from build123d import *

# Parameters (mm, degrees)
SKETCH1_R           = 2
SKETCH1_R_2         = 6
SKETCH1_R_3         = 3
BOSS_EXTRUDE1_DEPTH = 14
SKETCH2_R           = 6
SKETCH2_R_2         = 3
BOSS_EXTRUDE2_DEPTH = 38
SKETCH3_R           = 3
BOSS_EXTRUDE3_DEPTH = 12
SKETCH4_R           = 6
BOSS_EXTRUDE4_DEPTH = 22
CUT_EXTRUDE1_START  = -14
CUT_EXTRUDE1_DEPTH  = 14
CHAMFER1_SIZE       = 1
SKETCH6_R           = 2.5
CUT_EXTRUDE2_DEPTH  = 5
SKETCH7_R           = 1.5
CUT_EXTRUDE3_DEPTH  = 15


with BuildPart() as part:
    # Sketch1 → Boss-Extrude1 (new body)
    with BuildSketch(Plane(origin=(0, 0, 0), x_dir=(1, 0, 0), z_dir=(0, 1, 0))):
        with BuildLine():
            Line((5.196152423, -13), (-5.196152423, -13))
            ThreePointArc((-5.196152423, -13), (0, 14), (5.196152423, -13))
        make_face()
        with Locations(Location((-9, 0, 0), (0, 0, 270))):
            Circle(SKETCH1_R, mode=Mode.SUBTRACT)
        with Locations(Location((9, 0, 0), (0, 0, 270))):
            Circle(SKETCH1_R, mode=Mode.SUBTRACT)
        with Locations(Location((0, 5, 0), (0, 0, 270))):
            Circle(SKETCH1_R_2, mode=Mode.SUBTRACT)
        with Locations(Location((0, -8, 0), (0, 0, 270))):
            Circle(SKETCH1_R_3, mode=Mode.SUBTRACT)
    extrude(amount=BOSS_EXTRUDE1_DEPTH)

    # Sketch2 → Boss-Extrude2 (add)
    with BuildSketch(Plane(origin=(0, 14, 0), x_dir=(1, 0, 0), z_dir=(0, 1, 0))):
        with BuildLine():
            Line((-5.196152423, -13), (5.196152423, -13))
            ThreePointArc((5.196152423, -13), (0, 14), (-5.196152423, -13))
        make_face()
        with Locations(Location((0, 5, 0), (0, 0, 270))):
            Circle(SKETCH2_R, mode=Mode.SUBTRACT)
        with Locations(Location((0, -8, 0), (0, 0, 270))):
            Circle(SKETCH2_R_2, mode=Mode.SUBTRACT)
    extrude(amount=BOSS_EXTRUDE2_DEPTH)

    # Sketch3 → Boss-Extrude3 (add)
    with BuildSketch(Plane(origin=(0, 52, 0), x_dir=(1, 0, 0), z_dir=(0, 1, 0))):
        with BuildLine():
            Line((-5.196152423, -13), (5.196152423, -13))
            ThreePointArc((5.196152423, -13), (0, 14), (-5.196152423, -13))
        make_face()
        with Locations(Location((0, -8, 0), (0, 0, 270))):
            Circle(SKETCH3_R, mode=Mode.SUBTRACT)
    extrude(amount=BOSS_EXTRUDE3_DEPTH)

    # Sketch4 → Boss-Extrude4 (add)
    with BuildSketch(Plane(origin=(0, 64, 0), x_dir=(1, 0, 0), z_dir=(0, 1, 0))):
        with Locations(Location((0, 0, 0), (0, 0, 251.426650281))):
            Circle(SKETCH4_R)
    extrude(amount=BOSS_EXTRUDE4_DEPTH)

    # Sketch5 → Cut-Extrude1 (cut)
    with BuildSketch(Plane(origin=(0, 86, 0), x_dir=(1, 0, 0), z_dir=(0, 1, 0)).offset(CUT_EXTRUDE1_START)):
        with BuildLine():
            Line((5, 3.31662479), (5, -3.31662479))
            ThreePointArc((5, -3.31662479), (6, 0), (5, 3.31662479))
        make_face()
    extrude(amount=CUT_EXTRUDE1_DEPTH, mode=Mode.SUBTRACT)

    # Chamfer1
    chamfer1_edges = [part.edges().sort_by_distance(p)[0] for p in [
        (-4.759608727, 86, -3.653234836),
    ]]
    chamfer(chamfer1_edges, length=CHAMFER1_SIZE - 0.0001)  # a hair under: the kernel refuses the full size

    # Sketch6 → Cut-Extrude2 (cut)
    with BuildSketch(Plane.XY.offset(13)):
        with Locations((0, 31.800606355)):
            Circle(SKETCH6_R)
    extrude(amount=-CUT_EXTRUDE2_DEPTH, mode=Mode.SUBTRACT)

    # Sketch7 → Cut-Extrude3 (cut)
    with BuildSketch(Plane.XY.offset(13)):
        with Locations((0, 55)):
            Circle(SKETCH7_R)
    extrude(amount=-CUT_EXTRUDE3_DEPTH, mode=Mode.SUBTRACT)


solid = part.part
The model under review builds one solid part; all positions refer to its coordinate system, in mm. A direction names the side the tool comes from. Coordinates: 2 decimals unless noted, no trailing zeros. Write each loop counter-clockwise with the first axis right and the second up, starting at its lowest first coordinate (ties: lowest second). Pieces come first, ordered by that corner, then holes. Notation, with made-up numbers: (77, 13) - (94, 13) arc R22 cw to (94, 51) - close; hole circle Ø10 at (82, 77.25). An arc over 180 degrees is marked (long way). Answer as a JSON object with one key per item and string values. Group by question number.
1. Clearance check with flat-ended pins moving along their axes: pin 1 Ø0.9 at (x, y) = (0.5, 55) entering from +Z; pin 2 Ø11 at (x, z) = (0, -5) entering from -Y; pin 3 Ø8 at (x, y) = (-10, 34.5) entering from -Z. State where each tip first meets the part, or that it passes through.
2. Add section D-D (y = 39). Give the boundary of the cut face in (x, z), plus the area to 3 significant figures.
3. Add section B-B (z = 8). Give the boundary of the cut face in (x, y).
4. Mouldability with a two-part tool opening along Y and no side actions: class faces 1 (the face through (0, 52, -5)), 2 (the face through (1.386, 54.425, 11.816)), 3 (the face through (5, 79, 0)) as pulls with the +Y half, pulls with the -Y half, needs draft (parallel to the pull), parting line crosses it, or undercut.
5. Add section C-C (y = 55). Give the boundary of the cut face in (x, z), plus the area to 3 significant figures.
6. Add section A-A (x = 0). Give the number of separate pieces and of enclosed holes in the cut face, plus the area to 3 significant figures.
7. Machinability: for faces 4 (the face through (-5.928, 74.353, 0.929)), 5 (the face through (11, 7, 0)), 6 (the face through (1.386, 54.425, 1.753)), 7 (the face through (0, 86, 0)), which of the approach directions +Z, -Z, +X, -X, +Y, -Y give a long, thin tool a straight path to every point of the face, cutting with its end or side? Answer none if there is none.
8. To check wall thickness, follow probe 1 along Z at (x, y) = (-0.25, 37.5); probe 2 along X at (y, z) = (7.75, 0); probe 3 along Y at (x, z) = (0, 0). State the ranges of each line that lie inside material, in increasing order.
Findings:
{
 "1": {"pin 1": "z = -2", "pin 2": "y = 52", "pin 3": "z = -12.65"},
 "2": {"outline": "(-5.2, 13) arc R14 ccw (long way) to (5.2, 13) - close; hole circle Ø12 at (0, -5); hole circle Ø6 at (0, 8)", "area": "467 mm²"},
 "3": {"outline": "(-11.49, 0) - (-3, 0) - (-3, 64) - (-11.49, 64) - close; (3, 0) - (11.49, 0) - (11.49, 64) - (3, 64) - close"},
 "4": {"face 1": "pulls with the -Y half", "face 2": "undercut", "face 3": "needs draft"},
 "5": {"outline": "(-5.2, 13) arc R14 ccw (long way) to (5.2, 13) - (1.5, 13) - (1.5, 10.6) arc R3 cw to (1.5, 5.4) - (1.5, -2) - (-1.5, -2) - (-1.5, 5.4) arc R3 cw to (-1.5, 10.6) - (-1.5, 13) - close", "area": "553 mm²"},
 "6": {"separate pieces": "4", "enclosed holes": "0", "area": "946 mm²"},
 "7": {"face 4": "+Y", "face 5": "-Y", "face 6": "+Z", "face 7": "+Z, -Z, +X, -X, +Y"},
 "8": {"probe 1": "-14 to -10.99, 0.99 to 5.01, 10.99 to 13", "probe 2": "-14 to -11, -7 to -3.32, 3.32 to 7, 11 to 14", "probe 3": "52 to 53.5, 56.5 to 86"}
}
